Input: part model. Units: mm. Frame: model coordinates. Face numbers are marked on the shaded views. A direction names the side the tool comes from. Give positions to 0.01 mm unless a question says otherwise; leave off trailing zeros. Loops run counter-clockwise (first coordinate to the right, second up) from the corner with the lowest first, then second, coordinate; pieces in that order, holes last. Notation, with made-up numbers: (42, 31) -> (51, 31) arc R30 cw to (51, 68) -> close; hole circle Ø10 at (77.5, 36.25). An arc over 180 degrees is marked (long way). Answer as a JSON object with one key per item and string values.
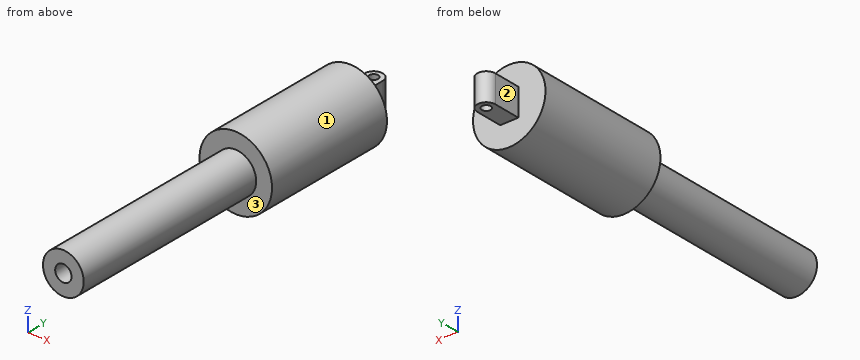
```python
from build123d import *

# Parameters (mm, degrees)
ESBO_O2_R                = 5
RESSALTO_EXTRUS_O1_DEPTH = 15


with BuildPart() as part:
    # Esboço1 → Revolução1 (revolve)
    with BuildSketch(Plane.XY):
        Polygon((0, 150), (40, 150), (40, 0), (22.5, 0), (22.5, -225), (9, -225), (9, 0), (0, 0), align=None)
    revolve(axis=Axis((0, 0, 0), (0, 1, 0)))

    # Esboço2 → Ressalto-extrusão1 (add, symmetric)
    with BuildSketch(Plane.XY):
        with BuildLine():
            Line((10, 150), (10, 180))
            ThreePointArc((10, 180), (0, 190), (-10, 180))
            Line((-10, 180), (-10, 150))
            Line((-10, 150), (10, 150))
        make_face()
        with Locations((0, 180)):
            Circle(ESBO_O2_R, mode=Mode.SUBTRACT)
    extrude(amount=RESSALTO_EXTRUS_O1_DEPTH, both=True)


solid = part.part
```
Q1. Section D-D, the plane z = -28. Return the cut outline in (x, y), then the cut area to 3 significant figures.
Evaluation:
{"outline": "(-28.57, 0) -> (28.57, 0) -> (28.57, 150) -> (-28.57, 150) -> close", "area": "8,570 mm2"}
Q2. Section C-C, the plane y = 82. Return the cut outline in (x, z).
Evaluation:
{"outline": "circle Ø80 at (0, 0)"}
Q3. Section B-B, the plane z = 0. Return the cut outline in (x, y).
Evaluation:
{"outline": "(-40, 0) -> (-22.5, 0) -> (-22.5, -225) -> (-9, -225) -> (-9, 0) -> (9, 0) -> (9, -225) -> (22.5, -225) -> (22.5, 0) -> (40, 0) -> (40, 150) -> (10, 150) -> (10, 180) arc R10 ccw to (-10, 180) -> (-10, 150) -> (-40, 150) -> close; hole circle Ø10 at (0, 180)"}
Q4. Ray query, line 1 along X through (y, z) = (-62.5, 0); line 2 along Y through (x, z) = (0, 0); line 3 along Y through (x, z) = (10, -23). Return the intervals inside material, ascending.
Evaluation:
{"line 1": "x = -22.5 to -9, 9 to 22.5", "line 2": "y = 0 to 175, 185 to 190", "line 3": "y = 0 to 150"}
Q5. Section A-A, the plane x = 0. Return the cut outline in (y, z).
Evaluation:
{"outline": "(-225, -22.5) -> (0, -22.5) -> (0, -40) -> (150, -40) -> (150, -15) -> (175, -15) -> (175, 15) -> (150, 15) -> (150, 40) -> (0, 40) -> (0, 22.5) -> (-225, 22.5) -> (-225, 9) -> (0, 9) -> (0, -9) -> (-225, -9) -> close; (185, -15) -> (190, -15) -> (190, 15) -> (185, 15) -> close"}
Q6. Access query for the marked faces 1, 2 and 3. Directions: +Z, -Z, +X, -X, +Y, -Y. A direction counts if a zero-diameter tool reaches every point of the face in a straight line with its end or side. Return the directions, or none.
Evaluation:
{"face 1": "+Y, -Y", "face 2": "+Z, -Z, -X, +Y", "face 3": "-Y"}
Q7. Pin query (flat end, axial travel): pin 1 (8 mm diameter, centred on x = 21.5, z = -8.5, fed in from -Y); pin 2 (2 mm diameter, centred on x = -22.5, y = 114, fed in from -Z); pin 3 (12 mm diameter, centred on x = 5.5, y = 105, fed in from -Z); pin 4 (22 mm diameter, centred on x = -0.5, y = 161.5, fed in from +Z). Return the tip coordinate at first contact, or that it passes through.
Evaluation:
{"pin 1": "stops at y = -225", "pin 2": "stops at z = -33.73", "pin 3": "stops at z = -40", "pin 4": "stops at z = 15"}
